from build123d import *

# Parameters (mm, degrees)
F2_R     = 0.75
F3_DEPTH = 70.001
F4_W     = 12
F4_H     = 20
F5_DEPTH = 25
F6_R     = 10
F7_DEPTH = 10
F8_SIZE  = 3


with BuildPart() as f1:
    # F0 (on Front) → F1 (revolve)
    with BuildSketch(Plane.XZ):
        Polygon((6.954034, 26.641815), (0, 26.641815), (0, 24.641815), (3, 24.641815), (5, 22.641815), (5, -43.358185), (12.3, -43.358185), (12.3, -39.858185), (16.3, -39.858185), align=None)
    revolve(axis=Axis((0, 0, 25.641815), (0, 0, 1)))

    # F2 (on face) → F3 (cut, through all)
    with BuildSketch(Plane.XY.offset(26.641815)):
        Circle(F2_R)
    extrude(amount=-F3_DEPTH, mode=Mode.SUBTRACT)

    # F4 (on Right) → F5 (cut)
    with BuildSketch(Plane.YZ):
        with Locations((0, -26.858185)):
            Rectangle(F4_W, F4_H)
    extrude(amount=-F5_DEPTH, mode=Mode.SUBTRACT)

    # F6 (on face) → F7 (cut)
    with BuildSketch(Plane(origin=(0, 0, -43.358185), x_dir=(1, 0, 0), z_dir=(0, 0, -1))):
        Circle(F6_R)
    extrude(amount=-F7_DEPTH, mode=Mode.SUBTRACT)

    # F8
    f8_edges = [f1.edges().sort_by_distance(p)[0] for p in [
        (-10, 0, -36.858185),
    ]]
    chamfer(f8_edges, length=F8_SIZE)


solid = f1.part
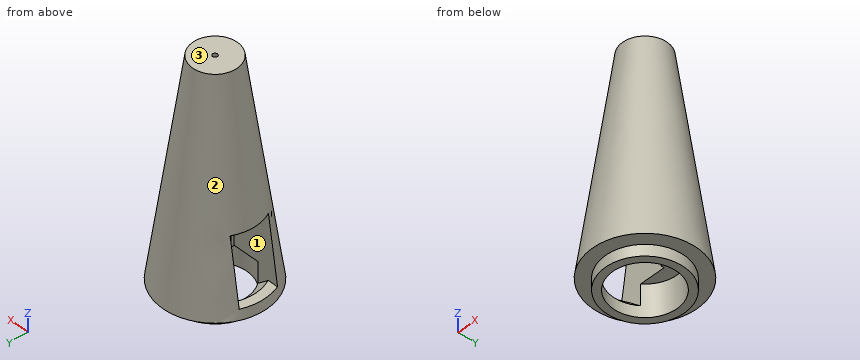
Could you check a few things on this model? Use its own coordinates, in mm. Face numbers are marked on the shaded views. Give positions to 0.01 mm unless a question says otherwise; leave off trailing zeros. Order: outer loops, then holes, each group sorted by start corner. A loop starts at its lowest first (then second) coordinate and runs counter-clockwise, first axis right, second up. Notation, with made-up numbers: (-11.5, 59) - (15.5, 59) arc R12 ccw to (15.5, 81) - close; hole circle Ø3 at (62, 13.25). An arc over 180 degrees is marked (long way). Return JSON: item names as keys, results as strings. Group by question number.
Q1. Suppose I cut it at B-B, the plane z = -16. Please give me the cut outline in (x, y), and give its area (3 significant figures).
Q2. Will these pins go through, and if not, where does the flat tip stop? pin 1 Ø4 at (y, z) = (-10.5, -25) entering from -X; pin 2 Ø5.5 at (x, y) = (3, -3) entering from -Z; pin 3 Ø12 at (x, z) = (-7, -23) entering from -Y.
Q3. Please list where these lines run through material, in increasing order: line 1 along X through (y, z) = (-0.5, -13.5); line 2 along X through (y, z) = (0, -16.5); line 3 along Y through (x, z) = (0, -36). Write a range as [from, to].
Q4. Thinking about a two-plate mould opening in Y: for the marked faces 1, 2 and 3, which applies, pulls with the +Y half, pulls with the -Y half, needs draft (parallel to the pull), parting line crosses it, or undercut?
Q5. Suppose I cut it at D-D, the plane z = 2.5. Please give me the cut outline in (x, y), and give its area (3 significant figures).
Q6. Suppose I cut it at A-A, the plane y = 0. Please give me the cut outline in (x, z).
Q7. Suppose I cut it at C-C, the plane z = -26. Please give me the cut outline in (x, y), and give its area (3 significant figures).
Resolved:
{
 "1": {"outline": "circle Ø25.89 at (0, 0); hole circle Ø10 at (0, 0)", "area": "448 mm2"},
 "2": {"pin 1": "stops at x = -11.43", "pin 2": "stops at z = -33.36", "pin 3": "stops at y = -14.27"},
 "3": {"line 1": "x = [-12.59, -4.97], [4.97, 12.59]", "line 2": "x = [-13.02, -5], [5, 13.02]", "line 3": "y = [-15.76, -10], [10, 15.76]"},
 "4": {"face 1": "undercut", "face 2": "parting line crosses it", "face 3": "needs draft"},
 "5": {"outline": "circle Ø20.69 at (0, 0); hole circle Ø10 at (0, 0)", "area": "258 mm2"},
 "6": {"outline": "(-16.3, -39.86) - (-12.3, -39.86) - (-12.3, -43.36) - (-10, -43.36) - (-10, -39.86) - (-13, -36.86) - (-15.88, -36.86) - close; (-13.07, -16.86) - (-5, -16.86) - (-5, 22.64) - (-3, 24.64) - (-0.75, 24.64) - (-0.75, 26.64) - (-6.95, 26.64) - close; (0.75, 24.64) - (3, 24.64) - (5, 22.64) - (5, -33.36) - (10, -33.36) - (10, -43.36) - (12.3, -43.36) - (12.3, -39.86) - (16.3, -39.86) - (6.95, 26.64) - (0.75, 26.64) - close"},
 "7": {"outline": "(-13.04, -6) arc R14.35 ccw (long way) to (-13.04, 6) - (0, 6) - (0, 5) arc R5 cw to (0, -5) - (0, -6) - close", "area": "441 mm2"}
}
